Autodesk Inventor part; units mm, degrees
ref_plane "YZ Plane" through (0, 0, 0) normal (1, 0, 0) x (0, 1, 0)
ref_plane "XZ Plane" through (0, 0, 0) normal (0, 1, 0) x (-1, 0, 0)
ref_plane "XY Plane" through (0, 0, 0) normal (0, 0, 1) x (1, 0, 0)
sketch "Sketch1" plane through (0, 0, 0) normal (0, 1, 0) x (-1, 0, 0)
  line L0 (0, 0) -> (76.2, 0)
  line L1 (76.2, 0) -> (76.2, -152.4)
  line L2 (76.2, -152.4) -> (0, -152.4)
  line L3 (0, -152.4) -> (0, 0)
  dimension "d0" = 76.2
  dimension "d1" = 152.4
extrude "Extrusion1" add sketch "Sketch1" along normal blind 9.525
sketch "Sketch2" plane through (0, 9.525, 0) normal (0, 1, 0) x (1, 0, 0)
  line L0 (-59.5312, 8.89) -> (-54.7688, 8.89)
  line L1 (-52.3875, 11.2712) -> (-52.3875, 59.5312)
  line L2 (-61.9125, 59.5312) -> (-61.9125, 11.2712)
  line L3 (-76.2, 152.4) -> (-76.2, 0)
  line L4 (-76.2, 0) -> (0, 0)
  arc A0 (-61.9125, 9.0487) -> (-61.7538, 8.89) centre (-61.7538, 9.0487) ccw
  arc A1 (-52.5462, 8.89) -> (-52.3875, 9.0487) centre (-52.5462, 9.0487) ccw
  arc A2 (-52.3875, 59.5312) -> (-52.5462, 59.69) centre (-52.5462, 59.5312) ccw
  arc A3 (-61.7538, 59.69) -> (-61.9125, 59.5312) centre (-61.7538, 59.5312) ccw
  line L5 (-60.6425, 59.69) -> (-53.6575, 59.69)
  line L6 (-53.6575, 59.69) -> (-53.6575, 116.84)
  line L7 (-60.6425, 116.84) -> (-60.6425, 59.69)
  line L8 (-52.5462, 59.69) -> (-53.6575, 59.69)
  line L9 (-60.6425, 59.69) -> (-61.7538, 59.69)
  line L10 (-68.2625, 116.84) -> (-46.0375, 116.84)
  line L11 (-42.8625, 113.665) -> (-42.8625, 88.9)
  line L12 (-46.0375, 85.725) -> (-68.2625, 85.725)
  line L13 (-71.4375, 88.9) -> (-71.4375, 113.665)
  arc A4 (-71.4375, 88.9) -> (-68.2625, 85.725) centre (-68.2625, 88.9) ccw
  arc A5 (-68.2625, 116.84) -> (-71.4375, 113.665) centre (-68.2625, 113.665) ccw
  arc A6 (-42.8625, 113.665) -> (-46.0375, 116.84) centre (-46.0375, 113.665) ccw
  arc A7 (-46.0375, 85.725) -> (-42.8625, 88.9) centre (-46.0375, 88.9) ccw
  arc A8 (-54.7688, 8.89) -> (-52.3875, 11.2712) centre (-54.7688, 11.2712) ccw
  arc A9 (-61.9125, 11.2712) -> (-59.5312, 8.89) centre (-59.5312, 11.2712) ccw
  point P0 (-61.9125, 8.89)
  point P1 (-52.3875, 69.85)
  point P2 (-52.3875, 8.89)
  point P3 (-61.9125, 69.85)
  point P4 (-57.15, 69.85)
  point P5 (-57.15, 132.715)
  point P6 (-71.4375, 116.84)
  point P7 (-42.8625, 85.725)
  point P8 (-42.8625, 116.84)
  point P9 (-71.4375, 85.725)
  point P10 (-57.15, 116.84)
  point P11 (-57.15, 8.89)
  point P12 (-57.15, 59.69)
  point P13 (-60.6425, 85.725)
  point P14 (-53.6575, 85.725)
  dimension "d22" = 0
  dimension "d28" = 0
  dimension "d36" = 26.035
  dimension "d37" = 50.8
  dimension "d41" = 9.525
  dimension "d47" = 2.3813
extrude "Extrusion2" cut sketch "Sketch2" against normal blind 0.254
sketch "Sketch3" plane through (0, 9.525, 0) normal (0, 1, 0) x (1, 0, 0)
  line L0 (-24.6057, 8.9288) -> (-19.8432, 8.9288)
  line L1 (-17.4619, 11.31) -> (-17.4619, 57.3087)
  line L2 (-26.9869, 57.3087) -> (-26.9869, 11.31)
  arc A0 (-26.9869, 11.31) -> (-24.6057, 8.9288) centre (-24.6057, 11.31) ccw
  arc A1 (-19.8432, 8.9288) -> (-17.4619, 11.31) centre (-19.8432, 11.31) ccw
  line L3 (-18.7319, 59.69) -> (-18.7319, 116.84)
  line L4 (-25.7169, 116.84) -> (-25.7169, 59.69)
  line L5 (0, 152.4) -> (-76.2, 152.4)
  line L6 (-32.5432, 116.84) -> (-11.9057, 116.84)
  line L7 (-8.7307, 113.665) -> (-8.7307, 88.9)
  line L8 (-11.9057, 85.725) -> (-32.5432, 85.725)
  line L9 (-35.7182, 88.9) -> (-35.7182, 113.665)
  line L10 (-46.0375, 85.725) -> (-53.6575, 85.725)
  arc A2 (-32.5432, 116.84) -> (-35.7182, 113.665) centre (-32.5432, 113.665) ccw
  arc A3 (-35.7182, 88.9) -> (-32.5432, 85.725) centre (-32.5432, 88.9) ccw
  arc A4 (-11.9057, 85.725) -> (-8.7307, 88.9) centre (-11.9057, 88.9) ccw
  arc A5 (-8.7307, 113.665) -> (-11.9057, 116.84) centre (-11.9057, 113.665) ccw
  line L11 (-17.4619, 57.3087) -> (-17.4619, 59.69)
  line L12 (-17.4619, 59.69) -> (-18.7319, 59.69)
  line L13 (-25.7169, 59.69) -> (-26.9869, 59.69)
  line L14 (-26.9869, 59.69) -> (-26.9869, 57.3087)
  point P0 (0, 0)
  point P1 (-26.9869, 8.9288)
  point P2 (-21.4307, 55.0791)
  point P3 (-22.2244, 132.715)
  point P4 (-8.7307, 85.725)
  point P5 (-35.7182, 85.725)
  point P6 (-22.2244, 116.84)
  point P7 (-49.8475, 85.725)
  point P8 (-25.7169, 85.725)
  point P9 (-18.7319, 116.84)
  point P10 (-18.7319, 85.725)
  point P11 (-25.1613, 59.69)
  point P12 (-22.2244, 8.9288)
  dimension "d12" = 9.525
  dimension "d13" = 2.3813
  dimension "d33" = 0
  dimension "d34" = 3.175
  dimension "d40" = 26.035
  dimension "d42" = 0
  dimension "d43" = 0
  dimension "d45" = 6.985
extrude "Extrusion3" cut sketch "Sketch3" against normal blind 0.889
properties part number "0p03_total_thickness"
The model under review builds one solid part; all positions refer to its coordinate system, in mm. A direction names the side the tool comes from. Round coordinates to 2 decimals unless told otherwise and drop trailing zeros. Use CSV: the item, a comma, the result in double quotes.
Q1. For faces 1 (the flat face through (-38, 5, 0)), 2 (the cylindrical face through (-9.64, 9.09, -115.89)), list the 3-axis set-ups (+Z, -Z, +X, -X, +Y, -Y) from which the entire face can be reached by the end or side of a thin tool; tool diameter is ignored.
Checks:
face 1,"+Z, +X, -X, +Y, -Y"
face 2,"+Y"
Q2. For pin 1 Ø8 at (x, z) = (-22.5, -50.5) entering from +Y, flat-tipped, find the tip position at first contact; note if it passes through.
Checks:
pin 1,"y = 8.64"
Q3. To check wall thickness, follow probe 1 along Y at (x, z) = (-29.5, -101); probe 2 along Y at (x, z) = (-47.5, -101.5). State the ranges of each line that lie inside material, in increasing order. Write a range as [from, to].
Checks:
probe 1,"[0, 8.64]"
probe 2,"[0, 9.27]"
Q4. Mouldability with a two-part tool opening along Z and no side actions: class faces 3 (the flat face through (0, 5, -77)), 4 (the flat face through (-39, 5, -152.4)), 5 (the cylindrical face through (-9.685, 9.087, -86.63)) as released by +Z, released by -Z, zero draft, split by the parting line, or undercut.
Checks:
face 3,"zero draft"
face 4,"released by -Z"
face 5,"undercut"
